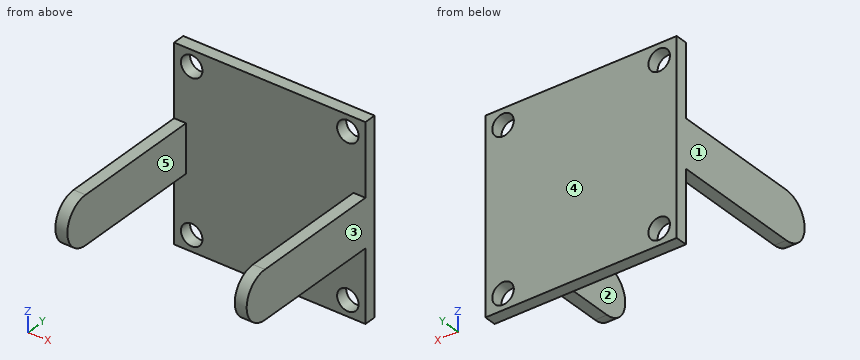
```python
from build123d import *

# Parameters (mm, degrees)
F0_W     = 101.6
F0_H     = 101.6
F1_DEPTH = 6.35
F2_R     = 5.715
F3_DEPTH = 6.35
F8_DEPTH = 6.35
F9_DEPTH = 6.35


with BuildPart() as f1:
    # F0 (on Front) → F1 (new body)
    with BuildSketch(Plane.XZ):
        Rectangle(F0_W, F0_H)
    extrude(amount=F1_DEPTH)

    # F2 (on Front) → F3 (cut)
    with BuildSketch(Plane.XZ):
        with Locations((-41.4617918432, 42.3875935376)):
            Circle(F2_R)
        with Locations((41.4617918432, 42.3875935376)):
            Circle(F2_R)
        with Locations((-41.4617918432, -42.3875935376)):
            Circle(F2_R)
        with Locations((41.4617918432, -42.3875935376)):
            Circle(F2_R)
    extrude(amount=F3_DEPTH, mode=Mode.SUBTRACT)

    # F7 (on offset) → F8 (join)
    with BuildSketch(Plane.YZ.offset(50.8)):
        with BuildLine():
            Line((0, -12.7), (0, 12.7))
            Line((0, 12.7), (-76.2, 12.7))
            ThreePointArc((-76.2, 12.7), (-88.9, 0), (-76.2, -12.7))
            Line((-76.2, -12.7), (0, -12.7))
        make_face()
    extrude(amount=-F8_DEPTH)

    # F5 (on offset) → F9 (join)
    with BuildSketch(Plane(origin=(-50.8, 0, 0), x_dir=(0, -1, 0), z_dir=(-1, 0, 0))):
        with BuildLine():
            Line((76.2, 12.7), (0, 12.7))
            Line((0, 12.7), (0, -12.7))
            Line((0, -12.7), (76.2, -12.7))
            ThreePointArc((76.2, -12.7), (88.9, 0), (76.2, 12.7))
        make_face()
    extrude(amount=-F9_DEPTH)


solid = f1.part
```
Model file for the job. Use its own axes, mm. Face numbers are marked on the shaded views. A direction names the side the tool comes from. Give positions to 0.01 mm unless a question says otherwise; leave off trailing zeros. Loops run counter-clockwise (first coordinate to the right, second up) from the corner with the lowest first, then second, coordinate; pieces in that order, holes last. Notation, with made-up numbers: (11.25, 79.5) - (25.25, 79.5) arc R30 ccw to (25.25, 118.5) - close; hole circle Ø6 at (20.25, 37.25). An arc over 180 degrees is marked (long way). One line per item, written item: value. Start each with the question number.
1. Slice it at B-B (z = 0). List the corners of the cut face in (x, y), plus the area to 3 significant figures.
2. Probe L1, parallel to Y at x = -40, z = -14; L2, parallel to X at y = -21.5, z = -2.5. List the from-to ranges inside material, lowest first. Write a range as from..to.
3. Slice it at A-A (y = -68.5). List the corners of the cut face in (x, z), plus the area to 3 significant figures.
4. Pin check, flat tips, straight feed: pin 1 (1.9 mm diameter, centred on x = 46.5, y = -46, fed in from -Z); pin 2 (3 mm diameter, centred on x = 49, y = -33, fed in from +Z); pin 3 (13 mm diameter, centred on x = -41.46, z = -42.39, fed in from -Y); pin 4 (6 mm diameter, centred on x = 7.5, z = -14.5, fed in from +Y). Stop position of each tip, or through.
5. Which spindle directions (+Z, -Z, +X, -X, +Y, -Y) get a long thin tool onto all of the face, cutting with end or side? Do the marked faces 4 and 5. Say none if no direction does.
6. Pull direction X, two halves, no side cores. Call the marked faces 1, 2 and 3: pulls with the +X half, pulls with the -X half, needs draft (parallel to the pull), parting line crosses it, or undercut.
7. Slice it at C-C (x = 15.5). List the corners of the cut face in (y, z), plus the area to 3 significant figures.
8. Slice it at D-D (y = -82.5). List the corners of the cut face in (x, z).
Solution:
1. outline: (-50.8, -88.9) - (-44.45, -88.9) - (-44.45, -6.35) - (44.45, -6.35) - (44.45, -88.9) - (50.8, -88.9) - (50.8, 0) - (-50.8, 0) - close
1. area: 1,690 mm^2
2. L1: y = -6.35..0
2. L2: x = -50.8..-44.45, 44.45..50.8
3. outline: (-50.8, -12.7) - (-44.45, -12.7) - (-44.45, 12.7) - (-50.8, 12.7) - close; (44.45, -12.7) - (50.8, -12.7) - (50.8, 12.7) - (44.45, 12.7) - close
3. area: 323 mm^2
4. pin 1: stops at z = -12.7
4. pin 2: stops at z = 12.7
4. pin 3: stops at y = -6.35
4. pin 4: stops at y = 0
5. face 4: +Z, -Z, +X, -X, +Y
5. face 5: +Z, -Z, -Y
6. face 1: pulls with the -X half
6. face 2: undercut
6. face 3: pulls with the +X half
7. outline: (-6.35, -50.8) - (0, -50.8) - (0, 50.8) - (-6.35, 50.8) - close
7. area: 645 mm^2
8. outline: (-50.8, -11.03) - (-44.45, -11.03) - (-44.45, 11.03) - (-50.8, 11.03) - close; (44.45, -11.03) - (50.8, -11.03) - (50.8, 11.03) - (44.45, 11.03) - close
